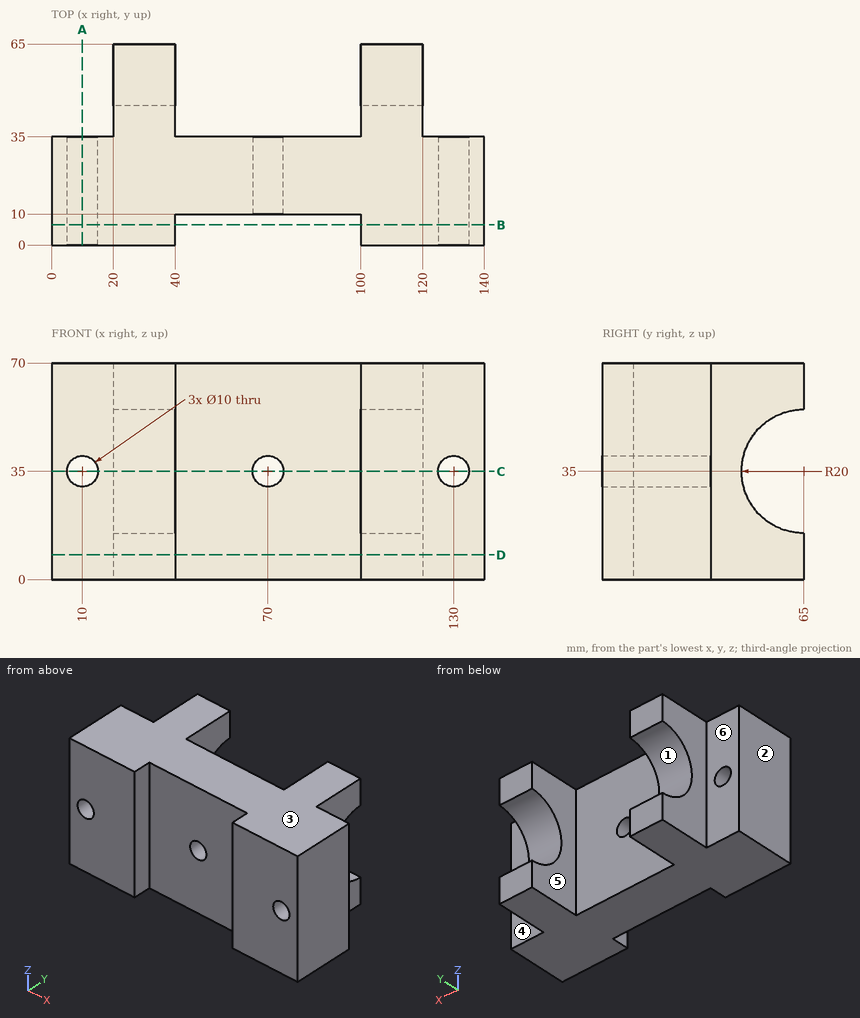
Part print with two shaded views. Sizes in mm from the minimum x, y, z corner. A direction names the side the tool comes from. Round coordinates to 2 decimals unless told otherwise and drop trailing zeros. Order: outer loops, then holes, each group sorted by start corner. A loop starts at its lowest first (then second) coordinate and runs counter-clockwise, first axis right, second up.
(1) Drill centre lines: line 1 (Z direction, x = 130, y = 14); line 2 (X direction, y = 50.5, z = 54); line 3 (Y direction, x = 122.5, z = 43.5). Where is each one in solid material? Low to high.
(2) 3-axis set-ups, long thin cutter, end or side, ignore diameter. For the marked faces 4, 5 and 6: which of +Z, -Z, +X, -X, +Y, -Y reach the whole face in a straight line?
(3) Band-saw the part on C-C (z = 35). List the corners of the cut face in (x, y), then the cut area to 3 significant figures.
(4) Band-saw the part on A-A (x = 10). List the corners of the cut face in (y, z), then the cut area to 3 significant figures.
(5) Pull direction Z, two halves, no side cores. Call the marked faces 1, 2 and 3: released by +Z, released by -Z, zero draft, split by the parting line, or undercut.
(6) Band-saw the part on D-D (z = 8). List the corners of the cut face in (x, y), then the cut area to 3 significant figures.
(7) Band-saw the part on B-B (y = 6.5). List the corners of the cut face in (x, z), then the cut area to 3 significant figures.
(8) Pin check, flat tips, straight feed: pin 1 (24 mm diameter, centred on y = 55.5, z = 36, fed in from +X); pin 2 (5 mm diameter, centred on x = 21, z = 12, fed in from -Y); pin 3 (9 mm diameter, centred on x = 10, z = 35, fed in from +Y); pin 4 (2 mm diameter, centred on x = 74.5, z = 50, fed in from -Y). Stop position of each tip, or through.
Verdict:
1. line 1: z = 0 to 30, 40 to 70
1. line 2: x = 20 to 40, 100 to 120
1. line 3: y = 0 to 35
2. face 4: +Z, -Z, +X, +Y
2. face 5: +Z, -Z, +Y
2. face 6: +Z, -Z, -X, +Y
3. outline: (0, 0) - (5, 0) - (5, 35) - (0, 35) - close; (15, 0) - (40, 0) - (40, 10) - (65, 10) - (65, 35) - (40, 35) - (40, 45) - (20, 45) - (20, 35) - (15, 35) - close; (75, 10) - (100, 10) - (100, 0) - (125, 0) - (125, 35) - (120, 35) - (120, 45) - (100, 45) - (100, 35) - (75, 35) - close; (135, 0) - (140, 0) - (140, 35) - (135, 35) - close
3. area: 3,750 mm2
4. outline: (0, 0) - (35, 0) - (35, 30) - (0, 30) - close; (0, 40) - (35, 40) - (35, 70) - (0, 70) - close
4. area: 2,100 mm2
5. face 1: undercut
5. face 2: zero draft
5. face 3: released by +Z
6. outline: (0, 0) - (40, 0) - (40, 10) - (100, 10) - (100, 0) - (140, 0) - (140, 35) - (120, 35) - (120, 65) - (100, 65) - (100, 35) - (40, 35) - (40, 65) - (20, 65) - (20, 35) - (0, 35) - close
6. area: 5,500 mm2
7. outline: (0, 0) - (40, 0) - (40, 70) - (0, 70) - close; (100, 0) - (140, 0) - (140, 70) - (100, 70) - close; hole circle Ø10 at (10, 35); hole circle Ø10 at (130, 35)
7. area: 5,440 mm2
8. pin 1: stops at x = 120
8. pin 2: stops at y = 0
8. pin 3: passes through
8. pin 4: stops at y = 10
